Study the drawing (mm; zero at the part's minimum x, y, z) and answer. Give positions to 0.01 mm unless a question says otherwise; leave off trailing zeros. Loops run counter-clockwise (first coordinate to the right, second up) from the corner with the lowest first, then second, coordinate; pieces in that order, holes last. Notation, with made-up numbers: M -1,21 L 18,21 A22 cw 18,33 Z; hole C 35,-34 d10. An arc over 180 degrees is marked long. Return JSON: item names as keys, results as strings.
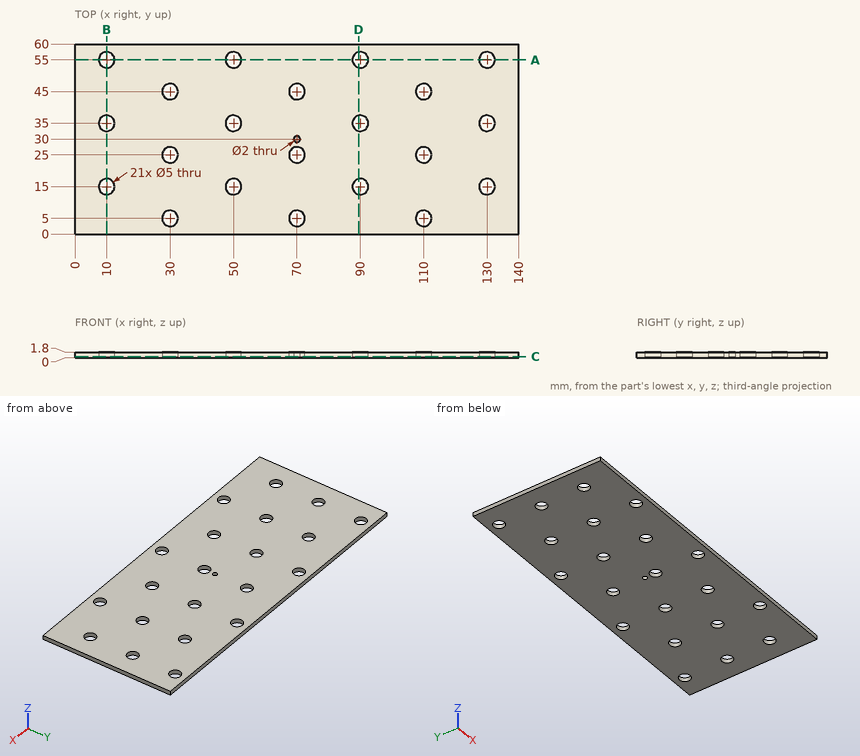
(1) The part is cut by section C-C (z = 0.4). Give the number of separate pieces and of enclosed holes in the cut face, and give its area (3 significant figures).
Values follow:
{"separate pieces": "1", "enclosed holes": "22", "area": "7,980 mm²"}
(2) Straight lines are drawn through the part: line 1 along Y through (x, z) = (70, 0.75); line 2 along Y through (x, z) = (30, 1.1); line 3 along Y through (x, z) = (50, 0.8). For each, find the intervals that lie inside material, in ascending order.
Values follow:
{"line 1": "0 to 2.5, 7.5 to 22.5, 27.5 to 29, 31 to 42.5, 47.5 to 60", "line 2": "0 to 2.5, 7.5 to 22.5, 27.5 to 42.5, 47.5 to 60", "line 3": "0 to 12.5, 17.5 to 32.5, 37.5 to 52.5, 57.5 to 60"}
(3) The part is cut by section A-A (y = 55). Determine the outline of the cut face in (x, z).
Values follow:
{"outline": "M 0,0 L 7.5,0 L 7.5,1.8 L 0,1.8 Z; M 12.5,0 L 47.5,0 L 47.5,1.8 L 12.5,1.8 Z; M 52.5,0 L 87.5,0 L 87.5,1.8 L 52.5,1.8 Z; M 92.5,0 L 127.5,0 L 127.5,1.8 L 92.5,1.8 Z; M 132.5,0 L 140,0 L 140,1.8 L 132.5,1.8 Z"}
(4) The part is cut by section D-D (x = 89.5). Determine the outline of the cut face in (y, z), and give its area (3 significant figures).
Values follow:
{"outline": "M 0,0 L 12.55,0 L 12.55,1.8 L 0,1.8 Z; M 17.45,0 L 32.55,0 L 32.55,1.8 L 17.45,1.8 Z; M 37.45,0 L 52.55,0 L 52.55,1.8 L 37.45,1.8 Z; M 57.45,0 L 60,0 L 60,1.8 L 57.45,1.8 Z", "area": "81.5 mm²"}
(5) The part is cut by section B-B (x = 10). Determine the outline of the cut face in (y, z), and give its area (3 significant figures).
Values follow:
{"outline": "M 0,0 L 12.5,0 L 12.5,1.8 L 0,1.8 Z; M 17.5,0 L 32.5,0 L 32.5,1.8 L 17.5,1.8 Z; M 37.5,0 L 52.5,0 L 52.5,1.8 L 37.5,1.8 Z; M 57.5,0 L 60,0 L 60,1.8 L 57.5,1.8 Z", "area": "81.0 mm²"}
